Part model, mm, in its own coordinate system. A direction names the side the tool comes from. Give positions to 0.01 mm unless a question says otherwise; leave off trailing zeros. Write each loop counter-clockwise with the first axis right and the second up, starting at its lowest first coordinate (ties: lowest second). Pieces come first, ordered by that corner, then holes. Notation, with made-up numbers: M 64,-9 L 79,-9 A13 cw 79,5 Z; hole C 73.25,4.5 d1. An arc over 180 degrees is marked long. Use a Markdown table: item, result.
Autodesk Inventor part; units mm, degrees
ref_plane "YZ Plane" through (0, 0, 0) normal (1, 0, 0) x (0, 1, 0)
ref_plane "XZ Plane" through (0, 0, 0) normal (0, 1, 0) x (-1, 0, 0)
ref_plane "XY Plane" through (0, 0, 0) normal (0, 0, 1) x (1, 0, 0)
sketch "Sketch1" plane through (0, 0, 0) normal (0, 0, 1) x (1, 0, 0)
  line L0 (0, 0) -> (139.7, 0)
  line L1 (139.7, 0) -> (139.7, 25.4)
  line L2 (139.7, 25.4) -> (0, 25.4)
  line L3 (0, 25.4) -> (0, 0)
  circle A0 centre (12.7, 12.7) radius 2.54
  circle A1 centre (25.4, 12.7) radius 4.445
  circle A2 centre (38.1, 12.7) radius 2.54
  circle A3 centre (50.8, 12.7) radius 2.54
  circle A4 centre (76.2, 12.7) radius 2.54
  circle A5 centre (88.9, 12.7) radius 4.445
  circle A6 centre (101.6, 12.7) radius 2.54
  circle A7 centre (127, 12.7) radius 4.445
  circle A8 centre (133.35, 6.35) radius 2.54
  circle A9 centre (120.65, 19.05) radius 2.54
  circle A10 centre (133.35, 19.05) radius 2.54
  circle A11 centre (120.65, 6.35) radius 2.54
  dimension "d0" = 139.7
  dimension "d1" = 25.4
  dimension "d9" = 5.08
  dimension "d11" = 8.89
  dimension "d13" = 5.08
  dimension "d15" = 5.08
  dimension "d17" = 5.08
  dimension "d19" = 8.89
  dimension "d21" = 5.08
  dimension "d23" = 8.89
  dimension "d39" = 5.08
  dimension "d42" = 5.08
  dimension "d43" = 5.08
  dimension "d44" = 5.08
extrude "Plate4" add sketch "Sketch1" along normal blind 1.5875
sketch "Sketch6" plane through (0, 26.9875, 3.175) normal (0, 1, 0) x (-1, 0, 0)
  line L0 (-139.7, 0) -> (0, 0)
  line L1 (0, 0) -> (0, 12.7)
  line L2 (0, 12.7) -> (-139.7, 12.7)
  line L3 (-139.7, 12.7) -> (-139.7, 0)
edge flange "Flange2" height 15.875 angle 90 thickness 1.5875 bend radius 1.5875 thickness toward (0, 1, 0) relief tear relief width 1.5875 relief depth 0.7937 edges at (69.85, 25.4, 1.5875) wall of the first edge with corners at (139.7, 26.9875, 3.175) (0, 26.9875, 3.175) (0, 26.9875, 15.875) (139.7, 26.9875, 15.875)
bend "Bend2"
corner "Corner2"
sketch "Sketch8" plane through (0, 28.575, 15.875) normal (0, 1, 0) x (1, 0, 0)
  line L0 (139.7, 12.7) -> (0, 12.7)
  line L1 (0, 12.7) -> (0, 6.35)
  line L2 (0, 0) -> (0, 12.7)
  line L3 (0, 6.35) -> (6.35, 6.35)
  circle A0 centre (6.35, 6.35) radius 2.54
  point P0 (0, 15.875)
  dimension "d69" = 6.35
  dimension "d70" = 5.08
extrude "Extrusion1" cut sketch "Sketch8" against normal blind 1.5875
equation "\"d58\" = Thickness"
equation "\"d59\" = BendReliefWidth"
equation "\"d60\" = BendReliefDepth"
equation "\"d61\" = MinimumRemnant"
equation "\"d62\" = TransitionRadius"
equation "\"d65\" = BendRadius"
equation "\"d66\" = CornerReliefSize"
equation "\"d67\" = GapSize"
equation "\"d68\" = JacobiRadiusSize"
equation "\"BendRadius\" = Thickness"
equation "\"BendReliefWidth\" = Thickness"
equation "\"BendReliefDepth\" = 0.5 * Thickness"
equation "\"CornerReliefSize\" = 4 * Thickness"
equation "\"MinimumRemnant\" = 2 * Thickness"
equation "\"TransitionRadius\" = BendRadius"
equation "\"JacobiRadiusSize\" = BendRadius"
equation "\"GapSize\" = Thickness"
properties part number "poly1"
1. Drill centre lines: L1, parallel to Y at x = 101, z = 9.75 (1 decimal); L2, parallel to Z at x = 121, y = 2.75; L3, parallel to Y at x = 88.9, z = 1.15 (3 decimals). Where is each one in solid material? Low to high.
Findings below:
| item | result |
|---|---|
| L1 | 27 to 28.6 |
| L2 | 0 to 1.59 |
| L3 | 0 to 8.255, 17.145 to 27.845 |
2. Drop flat-ended pins along their axis: P1, Ø1.5, axis at x = 97, y = 23.5, coming from the +Z side; P2, Ø3, axis at x = 112, z = 12, coming from the -Y side. Give the stop position or say it passes through.
Findings below:
| item | result |
|---|---|
| P1 | z = 1.59 |
| P2 | y = 26.99 |
3. Tool access for faces 4 (the cylindrical face through (53.223, 11.937, 0.783)), 5 (the flat face through (69, 26.988, 9)): list every direction of +Z, -Z, +X, -X, +Y, -Y with a clear straight run to the whole face (end or side of a thin tool).
Findings below:
| item | result |
|---|---|
| face 4 | +Z, -Z |
| face 5 | +Z, +X, -X, -Y |
4. Two-plate mould, pull along X, no slides. Class faces 1 (the cylindrical face through (12.15, 15.18, 0.78)), 2 (the flat face through (139.7, 17, 1)), 3 (the flat face through (69, 28.575, 10)): released by +X, released by -X, zero draft, split by the parting line, or undercut.
Findings below:
| item | result |
|---|---|
| face 1 | undercut |
| face 2 | released by +X |
| face 3 | zero draft |
5. Cut at A-A, the plane x = 133.35. State how many separate pieces and enclosed holes the cut face has, then the cut area to 3 significant figures.
Findings below:
| item | result |
|---|---|
| separate pieces | 3 |
| enclosed holes | 0 |
| area | 50.3 mm2 |
6. Cut at C-C, the plane y = 6.35. Give the cut face in (x, z).
Findings below:
| item | result |
|---|---|
| outline | M 0,0 L 118.11,0 L 118.11,1.59 L 0,1.59 Z; M 123.19,0 L 130.81,0 L 130.81,1.59 L 123.19,1.59 Z; M 135.89,0 L 139.7,0 L 139.7,1.59 L 135.89,1.59 Z |
